```python
from build123d import *

# Parameters (mm, degrees)
BOSS_EXTRU_1_DEPTH      = 15
BOSS_EXTRU_2_DEPTH      = 14
ESQUISSE3_W             = 4
ESQUISSE3_H             = 2
ENL_V_MAT_EXTRU_1_DEPTH = 10
BOSS_EXTRU_3_DEPTH      = 8
ESQUISSE6_R             = 1.5
ENL_V_MAT_EXTRU_2_DEPTH = 10
BOSS_EXTRU_4_DEPTH      = 14
ESQUISSE9_W             = 8
ESQUISSE9_H             = 8
ESQUISSE9_R             = 2.2
ESQUISSE9_R_2           = 2.3
BOSS_EXTRU_5_DEPTH      = 6


with BuildPart() as part:
    # Esquisse1 → Boss.-Extru.1 (new body)
    with BuildSketch(Plane.XY):
        Polygon((13, 0), (13, -9), (9, -13), (-9, -13), (-13, -9), (-13, 0), (-13, 9), (-9, 13), (0, 13), (9, 13), (13, 9), align=None)
        Polygon((7, 0), (7, -5), (5, -7), (-5, -7), (-7, -5), (-7, 0), (-7, 5), (-5, 7), (5, 7), (7, 5), align=None, mode=Mode.SUBTRACT)
    extrude(amount=BOSS_EXTRU_1_DEPTH)

    # Esquisse2 → Boss.-Extru.2 (add)
    with BuildSketch(Plane.XY.offset(15)):
        Polygon((-9, -13), (9, -13), (13, -9), (13, -1), (7, -1), (7, -5), (5, -7), (-5, -7), (-7, -5), (-7, -1), (-13, -1), (-13, -9), align=None)
    extrude(amount=BOSS_EXTRU_2_DEPTH)

    # Esquisse3 → Enlèv. mat.-Extru.1 (cut)
    with BuildSketch(Plane.XY.offset(15)):
        with Locations((-9, 0)):
            Rectangle(ESQUISSE3_W, ESQUISSE3_H)
        with Locations((9, 0)):
            Rectangle(ESQUISSE3_W, ESQUISSE3_H)
    extrude(amount=-ENL_V_MAT_EXTRU_1_DEPTH, mode=Mode.SUBTRACT)

    # Esquisse5 → Boss.-Extru.3 (add)
    with BuildSketch(Plane.XY.offset(29)):
        Polygon((-4, -1), (-7, -1), (-7, -5), (-5, -7), (-4, -7), align=None)
        Polygon((5, -7), (7, -5), (7, -1), (4, -1), (4, -7), align=None)
    extrude(amount=-BOSS_EXTRU_3_DEPTH)

    # Esquisse6 → Enlèv. mat.-Extru.2 (cut)
    with BuildSketch(Plane(origin=(0, -1, 0), x_dir=(1, 0, 0), z_dir=(0, 1, 0))):
        with Locations(Location((-7.5, -25, 0), (0, 0, 180))):
            Circle(ESQUISSE6_R)
        with Locations(Location((7.5, -25, 0), (0, 0, 180))):
            Circle(ESQUISSE6_R)
    extrude(amount=-ENL_V_MAT_EXTRU_2_DEPTH, mode=Mode.SUBTRACT)

    # Esquisse8 → Boss.-Extru.4 (add)
    with BuildSketch(Plane.XY.offset(29)):
        Polygon((-13, -9), (-9, -13), (-13, -13), align=None)
        Polygon((9, -13), (13, -13), (13, -9), align=None)
    extrude(amount=-BOSS_EXTRU_4_DEPTH)

    # Esquisse9 → Boss.-Extru.5 (add)
    # profile 1 of 2: a face of its own
    with BuildSketch(Plane.XZ.offset(13)):
        with Locations((-17, 19)):
            Rectangle(ESQUISSE9_W, ESQUISSE9_H)
        with Locations((-17, 19)):
            Circle(ESQUISSE9_R, mode=Mode.SUBTRACT)
    # profile 2 of 2: a face of its own
    with BuildSketch(Plane.XZ.offset(13)):
        with Locations((17, 19)):
            Rectangle(ESQUISSE9_W, ESQUISSE9_H)
        with Locations((17, 19)):
            Circle(ESQUISSE9_R_2, mode=Mode.SUBTRACT)
    extrude(amount=-BOSS_EXTRU_5_DEPTH)


solid = part.part
```
Could you check a few things on this model? Use its own coordinates, in mm. A direction names the side the tool comes from. Round coordinates to 2 decimals unless told otherwise and drop trailing zeros. Write each loop counter-clockwise with the first axis right and the second up, starting at its lowest first coordinate (ties: lowest second). Pieces come first, ordered by that corner, then holes. Notation, with made-up numbers: M 8.25,8 L 17.25,8 A29 cw 17.25,38 Z; hole C 38,-16.5 d2. An arc over 180 degrees is marked long. Answer in a Markdown table with one row per item. Add a question column.
Q1. Imagine slicing it at A-A (y = -4). Please give me the cut outline in (x, z), then the cut area to 3 significant figures.
Q2. Imagine slicing it at C-C (y = 2.75). Please give me the cut outline in (x, z), then the cut area to 3 significant figures.
Q3. Imagine slicing it at D-D (x = 2). Please give me the cut outline in (y, z), then the cut area to 3 significant figures.
Q4. On a 3-axis mill with a long thin cutter (end or side, diameter ignored), from which of +Z, -Z, +X, -X, +Y, -Y can I reach the whole of each face in a straight line? I mean faces 4 (the flat face through (5, -4, 21)), 5 (the flat face through (-11, 0, 10)), 6 (the flat face through (0, -7, 14)). Say none if no direction works.
Q5. Will these pins go through, and if not, where does the flat tip stop? pin 1 Ø0.9 at (x, z) = (-7, 25.5) entering from +Y; pin 2 Ø5 at (y, z) = (-1.5, 9.5) entering from -X; pin 3 Ø4 at (x, y) = (10.5, 6.5) entering from +Z.
Q6. If we mould it in two halves opening along Z, with no side actions, what happens to faces 1 (the flat face through (9, 0, 0)), 2 (the flat face through (-13, -2, 11)), 3 (the cylindrical face through (-7.305, -5.93, 26.487))? For each: +Z half, -Z half, draft (parallel to the pull), parting line (faces both ways), or undercut.
Q7. If I drill on line 1 (Z direction, x = -7.5, y = -3.5); line 2 (Y direction, x = 6, z = 13); line 3 (Z direction, x = 17, y = -9.2), over which ranges is the centre line in solid material (lowest first)? Write a range as from..to.
Q8. Imagine slicing it at B-B (z = 19). Please give me the cut outline in (x, y).
Values:
| question | item | result |
|---|---|---|
| 1 | outline | M -13,0 L -7,0 L -7,21 L -4,21 L -4,29 L -13,29 Z; M 4,21 L 7,21 L 7,0 L 13,0 L 13,29 L 4,29 Z; hole C -7.5,25 d3; hole C 7.5,25 d3 |
| 1 | area | 382 mm^2 |
| 2 | outline | M -13,0 L -7,0 L -7,15 L -13,15 Z; M 7,0 L 13,0 L 13,15 L 7,15 Z |
| 2 | area | 180 mm^2 |
| 3 | outline | M -13,0 L -7,0 L -7,29 L -13,29 Z; M 7,0 L 13,0 L 13,15 L 7,15 Z |
| 3 | area | 264 mm^2 |
| 4 | face 4 | -Z, +Y |
| 4 | face 5 | +Z |
| 4 | face 6 | -Z |
| 5 | pin 1 | y = -11 |
| 5 | pin 2 | x = -13 |
| 5 | pin 3 | z = 15 |
| 6 | face 1 | -Z half |
| 6 | face 2 | draft |
| 6 | face 3 | undercut |
| 7 | line 1 | 0..23.5, 26.5..29 |
| 7 | line 2 | -13..-6, 6..13 |
| 7 | line 3 | 15..16.7, 21.3..23 |
| 8 | outline | M -21,-13 L -19.2,-13 L -19.2,-7 L -21,-7 Z; M -14.8,-13 L 14.7,-13 L 14.7,-7 L 13,-7 L 13,-1 L 7,-1 L 7,-5 L 5,-7 L -5,-7 L -7,-5 L -7,-1 L -13,-1 L -13,-7 L -14.8,-7 Z; M 19.3,-13 L 21,-13 L 21,-7 L 19.3,-7 Z |
